Geometry check sheet. Reference: the model listing, model coordinates, mm. A direction names the side the tool comes from. Give positions to 0.01 mm unless a question says otherwise; leave off trailing zeros. Loops run counter-clockwise (first coordinate to the right, second up) from the corner with the lowest first, then second, coordinate; pieces in that order, holes last. Notation, with made-up numbers: (68, 3) - (87, 3) arc R16 cw to (87, 21) - close; hole circle Ø7 at (1, -2.5). An arc over 180 degrees is marked (long way). Use a Markdown table: item, result. Add a question column.
1. Cross-section at B-B on x = 77.5. Enter the section's corners in (y, z), and give its area (3 significant figures).
2. Depth check by flat-ended pin: P1, Ø7.5, axis at x = 82, y = 2, coming from the -Z side. Enter the tip coordinate at first touch or a pass-through.
3. Material ranges on L1, parallel to X at y = -3.5, z = -10; L2, parallel to X at y = 2.5, z = 11; L3, parallel to X at y = -15, z = -9, recorded low to high.
4. Set-up check for faces 5 (the cylindrical face through (-62, 3, -5)), 6 (the flat face through (-14, 0, -16)): record each of +Z, -Z, +X, -X, +Y, -Y from which the full face is reachable in a straight line by a thin tool's end or side.
5. Cross-section at C-C on x = 37. Enter the section's corners in (y, z), and give its area (3 significant figures).
6. Cross-section at A-A on z = -10. Enter the section's corners in (x, y), and give its area (3 significant figures).
7. Draft check along Y on faces 1 (the flat face through (-1, 16, 0)), 2 (the cylindrical face through (9.45, 3.37, 10.15)), 3 (the flat face through (93, 0, -16)), 4 (the flat face through (-1, -16, 0)). Enter one of: pulls with the +Y half, pulls with the -Y half, needs draft (parallel to the pull), parting line crosses it, or undercut.
from build123d import *

# Parameters (mm, degrees)
SKETCH2_W                                            = 190
SKETCH2_H                                            = 32
BOSS_EXTRUDE2_DEPTH                                  = 16
CHAMFER1_SIZE                                        = 2
SKETCH3_W                                            = 25
SKETCH3_H                                            = 4
CUT_EXTRUDE1_DEPTH                                   = 102.513545894
M12_TAPPED_HOLE1_D                                   = 10.2
M12_TAPPED_HOLE1_DEPTH                               = 24
M12_TAPPED_HOLE1_CSINK_D                             = 12.05
M12_TAPPED_HOLE1_CSINK_ANGLE                         = 90
M12_TAPPED_HOLE1_TIP                                 = 3.064389157
M4_TAPPED_HOLE1_D                                    = 3.3
M4_TAPPED_HOLE1_DEPTH                                = 11.5
M4_TAPPED_HOLE1_CSINK_D                              = 4.05
M4_TAPPED_HOLE1_CSINK_ANGLE                          = 90
M4_TAPPED_HOLE1_TIP                                  = 0.991420021
CSK_FOR_M10_COUNTERSUNK_FLAT_HEAD_SCREW1_D           = 6.5
CSK_FOR_M10_COUNTERSUNK_FLAT_HEAD_SCREW1_CSINK_D     = 13
CSK_FOR_M10_COUNTERSUNK_FLAT_HEAD_SCREW1_CSINK_ANGLE = 90
SKETCH13_R                                           = 3
CUT_EXTRUDE2_DEPTH                                   = 102.513545894
CSK_FOR_M4_COUNTERSUNK_FLAT_HEAD_SCREW1_D            = 1.5
CSK_FOR_M4_COUNTERSUNK_FLAT_HEAD_SCREW1_DEPTH        = 10
CSK_FOR_M4_COUNTERSUNK_FLAT_HEAD_SCREW1_CSINK_D      = 4
CSK_FOR_M4_COUNTERSUNK_FLAT_HEAD_SCREW1_CSINK_ANGLE  = 90
CSK_FOR_M4_COUNTERSUNK_FLAT_HEAD_SCREW1_TIP          = 0.450645464
M4_TAPPED_HOLE2_D                                    = 3.3
M4_TAPPED_HOLE2_DEPTH                                = 16
M4_TAPPED_HOLE2_CSINK_D                              = 4
M4_TAPPED_HOLE2_CSINK_ANGLE                          = 90
M4_TAPPED_HOLE2_TIP                                  = 0.991420021
SKETCH19_R                                           = 3
CUT_EXTRUDE3_DEPTH                                   = 102.51354591


with BuildPart() as part:
    # Sketch2 → Boss-Extrude2 (new, symmetric)
    with BuildSketch(Plane.XY):
        Rectangle(SKETCH2_W, SKETCH2_H)
    extrude(amount=BOSS_EXTRUDE2_DEPTH, both=True)

    # Chamfer1
    chamfer1_edges = [part.edges().sort_by_distance(p)[0] for p in [
        (-95, 0, 16),
        (95, 0, 16),
        (-95, 0, -16),
    ]]
    chamfer(chamfer1_edges, length=CHAMFER1_SIZE)

    # Sketch3 → Cut-Extrude1 (cut, through all)
    with BuildSketch(Plane(origin=(0, 16, 0), x_dir=(1, 0, 0), z_dir=(0, 1, 0))):
        with Locations((79.5, 14)):
            Rectangle(SKETCH3_W, SKETCH3_H)
    extrude(amount=-CUT_EXTRUDE1_DEPTH, mode=Mode.SUBTRACT)

    # M12 Tapped Hole1
    with Locations(Plane(origin=(0, 16, 0), x_dir=(1, 0, 0), z_dir=(0, 1, 0))):
        with Locations((-63, 0), (11, 0)):
            CounterSinkHole(M12_TAPPED_HOLE1_D / 2, M12_TAPPED_HOLE1_CSINK_D / 2, depth=M12_TAPPED_HOLE1_DEPTH, counter_sink_angle=M12_TAPPED_HOLE1_CSINK_ANGLE)
            with Locations((0, 0, -(M12_TAPPED_HOLE1_DEPTH + M12_TAPPED_HOLE1_TIP / 2))):  # 118° drill point
                Cone(0, M12_TAPPED_HOLE1_D / 2, M12_TAPPED_HOLE1_TIP, mode=Mode.SUBTRACT)

    # M4 Tapped Hole1
    with Locations(Plane.XY.offset(16)):
        with Locations((-63.030813748, 4), (10.974374685, 4)):
            CounterSinkHole(M4_TAPPED_HOLE1_D / 2, M4_TAPPED_HOLE1_CSINK_D / 2, depth=M4_TAPPED_HOLE1_DEPTH, counter_sink_angle=M4_TAPPED_HOLE1_CSINK_ANGLE)
            with Locations((0, 0, -(M4_TAPPED_HOLE1_DEPTH + M4_TAPPED_HOLE1_TIP / 2))):  # 118° drill point
                Cone(0, M4_TAPPED_HOLE1_D / 2, M4_TAPPED_HOLE1_TIP, mode=Mode.SUBTRACT)

    # CSK for M10 Countersunk Flat Head Screw1 (through all)
    with Locations(Plane.XY.offset(16)):
        with Locations((77.5, 4)):
            CounterSinkHole(CSK_FOR_M10_COUNTERSUNK_FLAT_HEAD_SCREW1_D / 2, CSK_FOR_M10_COUNTERSUNK_FLAT_HEAD_SCREW1_CSINK_D / 2, counter_sink_angle=CSK_FOR_M10_COUNTERSUNK_FLAT_HEAD_SCREW1_CSINK_ANGLE)

    # Sketch13 → Cut-Extrude2 (cut, through all)
    with BuildSketch(Plane.XY.offset(16)):
        with Locations((-87.030813748, 6)):
            Circle(SKETCH13_R)
    extrude(amount=-CUT_EXTRUDE2_DEPTH, mode=Mode.SUBTRACT)

    # CSK for M4 Countersunk Flat Head Screw1
    with Locations(Plane(origin=(0, 16, 0), x_dir=(1, 0, 0), z_dir=(0, 1, 0))):
        with Locations((-87, 0)):
            CounterSinkHole(CSK_FOR_M4_COUNTERSUNK_FLAT_HEAD_SCREW1_D / 2, CSK_FOR_M4_COUNTERSUNK_FLAT_HEAD_SCREW1_CSINK_D / 2, depth=CSK_FOR_M4_COUNTERSUNK_FLAT_HEAD_SCREW1_DEPTH, counter_sink_angle=CSK_FOR_M4_COUNTERSUNK_FLAT_HEAD_SCREW1_CSINK_ANGLE)
            with Locations((0, 0, -(CSK_FOR_M4_COUNTERSUNK_FLAT_HEAD_SCREW1_DEPTH + CSK_FOR_M4_COUNTERSUNK_FLAT_HEAD_SCREW1_TIP / 2))):  # 118° drill point
                Cone(0, CSK_FOR_M4_COUNTERSUNK_FLAT_HEAD_SCREW1_D / 2, CSK_FOR_M4_COUNTERSUNK_FLAT_HEAD_SCREW1_TIP, mode=Mode.SUBTRACT)

    # M4 Tapped Hole2
    with Locations(Plane(origin=(0, 16, 0), x_dir=(1, 0, 0), z_dir=(0, 1, 0))):
        with Locations((-43, 0)):
            CounterSinkHole(M4_TAPPED_HOLE2_D / 2, M4_TAPPED_HOLE2_CSINK_D / 2, depth=M4_TAPPED_HOLE2_DEPTH, counter_sink_angle=M4_TAPPED_HOLE2_CSINK_ANGLE)
            with Locations((0, 0, -(M4_TAPPED_HOLE2_DEPTH + M4_TAPPED_HOLE2_TIP / 2))):  # 118° drill point
                Cone(0, M4_TAPPED_HOLE2_D / 2, M4_TAPPED_HOLE2_TIP, mode=Mode.SUBTRACT)

    # Sketch19 → Cut-Extrude3 (cut, through all)
    with BuildSketch(Plane(origin=(0, 16, 0), x_dir=(1, 0, 0), z_dir=(0, 1, 0))):
        with Locations(Location((-37, 10, 0), (0, 0, 270))):
            Circle(SKETCH19_R)
        with Locations(Location((37, 10, 0), (0, 0, 270))):
            Circle(SKETCH19_R)
    extrude(amount=-CUT_EXTRUDE3_DEPTH, mode=Mode.SUBTRACT)


solid = part.part
Values found:
| question | item | result |
|---|---|---|
| 1 | outline | (-16, -12) - (0.75, -12) - (0.75, 12.75) - (-2.5, 16) - (-16, 16) - close; (7.25, -12) - (16, -12) - (16, 16) - (10.5, 16) - (7.25, 12.75) - close |
| 1 | area | 703 mm2 |
| 2 | P1 | stops at z = -12 |
| 3 | L1 | x = -95 to -40, -34 to 34, 40 to 95 |
| 3 | L2 | x = -95 to -63.72, -62.34 to 10.29, 11.66 to 74.62, 80.38 to 95 |
| 3 | L3 | x = -95 to -39.83, -34.17 to 34.17, 39.83 to 95 |
| 4 | face 5 | +Y |
| 4 | face 6 | -Z, +X, -X, +Y, -Y |
| 5 | outline | (-16, -16) - (16, -16) - (16, -13) - (-16, -13) - close; (-16, -7) - (16, -7) - (16, 16) - (-16, 16) - close |
| 5 | area | 832 mm2 |
| 6 | outline | (-95, -16) - (-40, -16) - (-40, 16) - (-95, 16) - close; (-34, -16) - (34, -16) - (34, 16) - (-34, 16) - close; (40, -16) - (95, -16) - (95, 16) - (40, 16) - close; hole circle Ø6 at (-87.03, 6); hole circle Ø6.5 at (77.5, 4) |
| 6 | area | 5,630 mm2 |
| 7 | face 1 | pulls with the +Y half |
| 7 | face 2 | undercut |
| 7 | face 3 | needs draft |
| 7 | face 4 | pulls with the -Y half |
